Check sheet for the modelled part. Datum: model origin and axes. Units: mm. Give positions to 0.01 mm unless a question says otherwise; leave off trailing zeros. Order: outer loops, then holes, each group sorted by start corner. A loop starts at its lowest first (then second) coordinate and runs counter-clockwise, first axis right, second up.
Autodesk Inventor part; units mm, degrees
ref_plane "YZ Plane" through (0, 0, 0) normal (1, 0, 0) x (0, 1, 0)
ref_plane "XZ Plane" through (0, 0, 0) normal (0, 1, 0) x (-1, 0, 0)
ref_plane "XY Plane" through (0, 0, 0) normal (0, 0, 1) x (1, 0, 0)
sketch "Sketch1" plane through (0, 0, 0) normal (0, 1, 0) x (-1, 0, 0)
  arc A0 (210.5939, -215.9) -> (210.5939, 215.9) centre (0, 0) ccw
  line L0 (470.9439, 215.9) -> (470.9439, -215.9)
  line L1 (470.9439, 215.9) -> (407.4439, 215.9)
  line L2 (407.4439, 215.9) -> (407.4439, 95.25)
  line L3 (407.4439, 95.25) -> (331.2439, 95.25)
  line L4 (331.2439, 95.25) -> (331.2439, 215.9)
  line L5 (470.9439, -215.9) -> (407.4439, -215.9)
  line L6 (407.4439, -215.9) -> (407.4439, -95.25)
  line L7 (407.4439, -95.25) -> (331.2439, -95.25)
  line L8 (331.2439, -95.25) -> (331.2439, -215.9)
  line L9 (331.2439, 215.9) -> (210.5939, 215.9)
  line L10 (331.2439, -215.9) -> (210.5939, -215.9)
  circle A1 centre (458.2439, 203.2) radius 2.4892
  circle A2 centre (445.5439, 203.2) radius 2.4892
  circle A3 centre (432.8439, 203.2) radius 2.4892
  circle A4 centre (420.1439, 203.2) radius 2.4892
  circle A5 centre (318.5439, 203.2) radius 2.4892
  circle A6 centre (305.8439, 203.2) radius 2.4892
  circle A7 centre (293.1439, 203.2) radius 2.4892
  circle A8 centre (280.4439, 203.2) radius 2.4892
  circle A9 centre (267.7439, 203.2) radius 2.4892
  circle A10 centre (255.0439, 203.2) radius 2.4892
  circle A11 centre (242.3439, 203.2) radius 2.4892
  circle A12 centre (229.6439, 203.2) radius 2.4892
  line L11 (597.6164, 0) -> (168.2721, 0) construction
  circle A13 centre (458.2439, -203.2) radius 2.4892
  circle A14 centre (445.5439, -203.2) radius 2.4892
  circle A15 centre (432.8439, -203.2) radius 2.4892
  circle A16 centre (420.1439, -203.2) radius 2.4892
  circle A17 centre (318.5439, -203.2) radius 2.4892
  circle A18 centre (305.8439, -203.2) radius 2.4892
  circle A19 centre (293.1439, -203.2) radius 2.4892
  circle A20 centre (280.4439, -203.2) radius 2.4892
  circle A21 centre (267.7439, -203.2) radius 2.4892
  circle A22 centre (255.0439, -203.2) radius 2.4892
  circle A23 centre (242.3439, -203.2) radius 2.4892
  circle A24 centre (229.6439, -203.2) radius 2.4892
  dimension "d0" = 603.2002
  dimension "d1" = 431.8
  dimension "d2" = 63.5
  dimension "d3" = 120.65
  dimension "d4" = 76.2
  dimension "d5" = 63.5
  dimension "d6" = 120.65
  dimension "d7" = 76.2
  dimension "d8" = 120.65
  dimension "d9" = 120.65
  dimension "d10" = 4.9784
  dimension "d11" = 12.7
  dimension "d12" = 12.7
  dimension "d15" = 12.7
  dimension "d20" = 4.9784
  dimension "d21" = 12.7
  dimension "d22" = 12.7
  dimension "d25" = 12.7
  dimension "d30" = 12.7
extrude "Extrusion1" add sketch "Sketch1" along normal blind 6.35
sketch "Sketch2" plane through (0, 6.35, 0) normal (0, 1, 0) x (1, 0, 0)
  line L0 (-407.4439, -215.9) -> (-407.4439, -95.25)
  line L1 (-407.4439, -95.25) -> (-331.2439, -95.25)
  line L2 (-331.2439, -95.25) -> (-331.2439, -215.9)
  line L3 (-331.2439, -215.9) -> (-210.5939, -215.9)
  arc A0 (-210.5939, 215.9) -> (-210.5939, -215.9) centre (0, 0) ccw
  line L4 (-210.5939, 215.9) -> (-331.2439, 215.9)
  line L5 (-331.2439, 215.9) -> (-331.2439, 95.25)
  line L6 (-331.2439, 95.25) -> (-407.4439, 95.25)
  line L7 (-407.4439, 95.25) -> (-407.4439, 215.9)
  line L8 (-407.4439, 215.9) -> (-470.9439, 215.9)
  line L9 (-470.9439, 215.9) -> (-470.9439, -215.9)
  line L10 (-470.9439, -215.9) -> (-407.4439, -215.9)
  circle A1 centre (-305.8439, 203.2) radius 2.4892
  circle A2 centre (-458.2439, 203.2) radius 2.4892
  circle A3 centre (-432.8439, 203.2) radius 2.4892
  circle A4 centre (-420.1439, 203.2) radius 2.4892
  circle A5 centre (-305.8439, -203.2) radius 2.4892
  circle A6 centre (-318.5439, -203.2) radius 2.4892
  circle A7 centre (-420.1439, -203.2) radius 2.4892
  circle A8 centre (-432.8439, -203.2) radius 2.4892
  circle A9 centre (-445.5439, -203.2) radius 2.4892
  circle A10 centre (-458.2439, -203.2) radius 2.4892
  circle A11 centre (-445.5439, 203.2) radius 2.4892
  circle A12 centre (-318.5439, 203.2) radius 2.4892
  circle A13 centre (-293.1439, 203.2) radius 2.4892
  circle A14 centre (-280.4439, 203.2) radius 2.4892
  circle A15 centre (-267.7439, 203.2) radius 2.4892
  circle A16 centre (-255.0439, 203.2) radius 2.4892
  circle A17 centre (-242.3439, 203.2) radius 2.4892
  circle A18 centre (-229.6439, 203.2) radius 2.4892
  circle A19 centre (-229.6439, -203.2) radius 2.4892
  circle A20 centre (-242.3439, -203.2) radius 2.4892
  circle A21 centre (-255.0439, -203.2) radius 2.4892
  circle A22 centre (-267.7439, -203.2) radius 2.4892
  circle A23 centre (-280.4439, -203.2) radius 2.4892
  circle A24 centre (-293.1439, -203.2) radius 2.4892
  line L11 (-470.9439, -215.9) -> (-255.0439, -215.9)
  line L12 (-255.0439, -215.9) -> (-244.8331, 215.9)
  point P0 (-253.7918, -162.9489)
  point P1 (-245.8059, 174.7629)
  dimension "d33" = 215.9
extrude "Extrusion2" add sketch "Sketch2" against normal up to surface (6.35 mm away) contours A0 L12
extrude "Extrusion3" cut sketch "Sketch2" against normal blind 25.4 contours L12 A21 A0 L3 | L12 A21 | L12 L4 A0 picked at (-254.0374, -203.0094)
sketch "Sketch3" plane through (0, 6.35, 0) normal (0, 1, 0) x (1, 0, 0)
  line L0 (-254.6854, -200.7368) -> (-244.8331, 215.9)
  line L1 (-244.8331, 215.9) -> (-331.2439, 215.9)
  line L2 (-331.2439, 215.9) -> (-331.2439, 95.25)
  line L3 (-331.2439, 95.25) -> (-407.4439, 95.25)
  line L4 (-407.4439, 95.25) -> (-407.4439, 215.9)
  line L5 (-407.4439, 215.9) -> (-470.9439, 215.9)
  line L6 (-470.9439, 215.9) -> (-470.9439, -215.9)
  line L7 (-470.9439, -215.9) -> (-407.4439, -215.9)
  line L8 (-407.4439, -215.9) -> (-407.4439, -95.25)
  line L9 (-407.4439, -95.25) -> (-331.2439, -95.25)
  line L10 (-331.2439, -95.25) -> (-331.2439, -215.9)
  line L11 (-331.2439, -215.9) -> (-255.0439, -215.9)
  line L12 (-255.0439, -215.9) -> (-254.8022, -205.6774)
  arc A0 (-254.6854, -200.7368) -> (-254.8022, -205.6774) centre (-255.0439, -203.2) ccw
  circle A1 centre (-305.8439, 203.2) radius 2.4892
  circle A2 centre (-458.2439, 203.2) radius 2.4892
  circle A3 centre (-432.8439, 203.2) radius 2.4892
  circle A4 centre (-420.1439, 203.2) radius 2.4892
  circle A5 centre (-305.8439, -203.2) radius 2.4892
  circle A6 centre (-318.5439, -203.2) radius 2.4892
  circle A7 centre (-420.1439, -203.2) radius 2.4892
  circle A8 centre (-432.8439, -203.2) radius 2.4892
  circle A9 centre (-445.5439, -203.2) radius 2.4892
  circle A10 centre (-458.2439, -203.2) radius 2.4892
  circle A11 centre (-445.5439, 203.2) radius 2.4892
  circle A12 centre (-318.5439, 203.2) radius 2.4892
  circle A13 centre (-293.1439, 203.2) radius 2.4892
  circle A14 centre (-280.4439, 203.2) radius 2.4892
  circle A15 centre (-267.7439, 203.2) radius 2.4892
  circle A16 centre (-255.0439, 203.2) radius 2.4892
  circle A17 centre (-267.7439, -203.2) radius 2.4892
  circle A18 centre (-280.4439, -203.2) radius 2.4892
  circle A19 centre (-293.1439, -203.2) radius 2.4892
  point P0 (0, 0)
extrude "Extrusion4" cut sketch "Sketch3" against normal blind 3.175
properties part number "Polycarbonate-Note-Intakaur-Cover" material "Polycarbonate, Smoke"
Q1. Sectioned sample at D-D, the plane z = -106.5. Record the cut outline in (x, y) (3 decimals).
Q2. Sectioned sample at B-B, the plane y = 2.55. Count the separate pieces of the cut face and the enclosed holes in it, plus the area to 3 significant figures.
Q3. Go/stop test with flat-tipped pins: P1, Ø1.6, axis at y = 2, z = -154, coming from the +X side; P2, Ø10, axis at x = -272, z = 147.5, coming from the -Y side; P3, Ø1.5, axis at x = -339, y = 2.5, coming from the +Z side; P4, Ø1.6, axis at x = -379.5, y = 1, coming from the -Z side. Record where each tip stops, or that it passes through.
Q4. Sectioned sample at C-C, the plane x = -341. Record the cut outline in (y, z) (3 decimals), plus the area to 3 significant figures.
Q5. Material ranges on line 1 (Z direction, x = -319, y = 1.8); line 2 (Z direction, x = -407, y = 2.8); line 3 (Z direction, x = -304.5, y = 2.25), recorded low to high.
Q6. Sectioned sample at A-A, the plane z = -165. Record the cut outline in (x, y) (3 decimals).
Filled in:
1. outline: (-470.944, 0) - (-407.444, 0) - (-407.444, 3.175) - (-470.944, 3.175) - close; (-331.244, 0) - (-247.42, 0) - (-247.42, 3.175) - (-331.244, 3.175) - close
2. separate pieces: 1
2. enclosed holes: 19
2. area: 76,700 mm2
3. P1: stops at x = -246.28
3. P2: stops at y = 0
3. P3: stops at z = 95.25
3. P4: stops at z = -95.25
4. outline: (0, -95.25) - (3.175, -95.25) - (3.175, 95.25) - (0, 95.25) - close
4. area: 605 mm2
5. line 1: z = -215.9 to -205.65, -200.75 to 200.75, 205.65 to 215.9
5. line 2: z = -95.25 to 95.25
5. line 3: z = -215.9 to -205.3, -201.1 to 201.1, 205.3 to 215.9
6. outline: (-470.944, 0) - (-407.444, 0) - (-407.444, 3.175) - (-470.944, 3.175) - close; (-331.244, 0) - (-246.037, 0) - (-246.037, 3.175) - (-331.244, 3.175) - close
